Can you work these out from the drawing? Everything is in mm from the part's minimum corner. A direction names the side the tool comes from. Coordinates: 2 decimals unless noted, no trailing zeros. Write each loop counter-clockwise with the first axis right and the second up, starting at its lowest first coordinate (ties: lowest second). Pieces come first, ordered by that corner, then holes. Notation, with made-up numbers: (12, 43.25) -> (64, 43.25) arc R16 ccw to (64, 71.25) -> close; hole circle Ø4 at (4.25, -36). An arc over 180 degrees is marked (long way). Use CSV: the item, a comma, the result in double quotes. Start each with the question number.
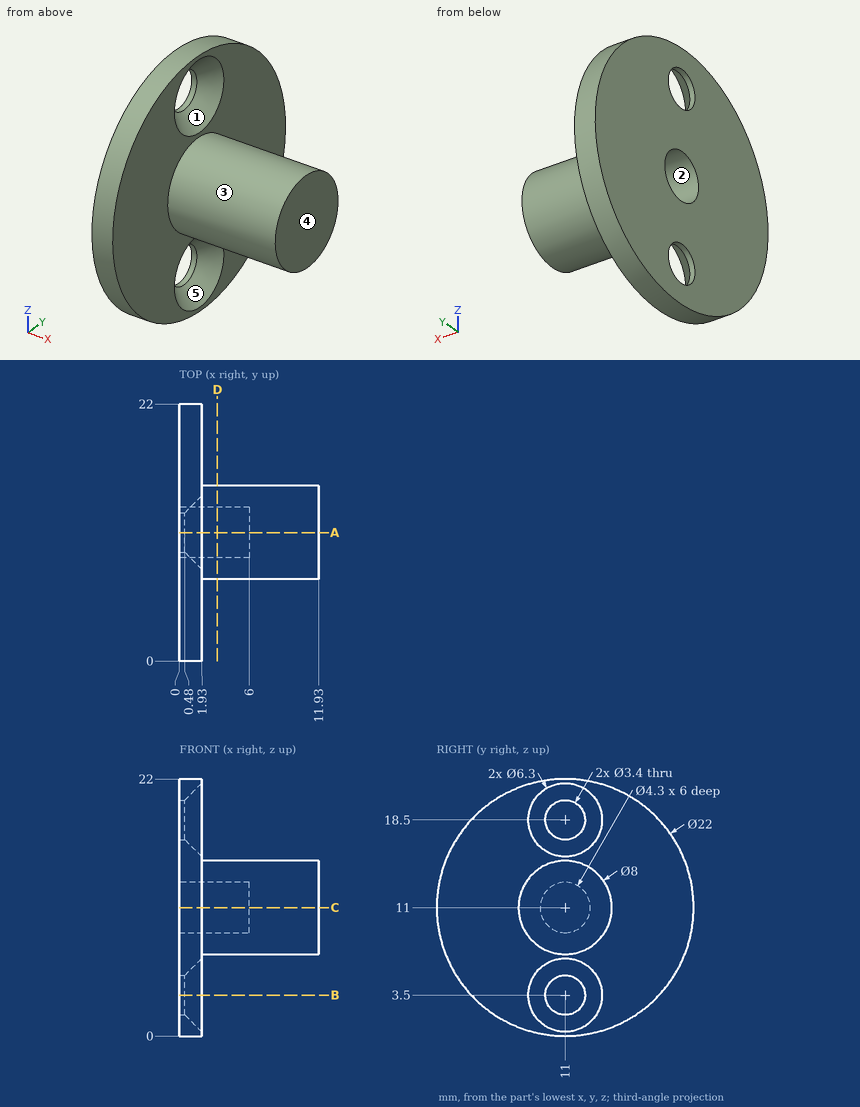
Item 1: Which directions (+Z, -Z, +X, -X, +Y, -Y) give clear straight access to the entire face, cutting with the end or side of a thin tool? Please do the marked faces 1 and 2.
Item 2: I want a section at C-C on z = 11. Please give me the cut outline in (x, y), then the cut area to 3 significant figures.
Item 3: I want a section at B-B on z = 3.5. Please give me the cut outline in (x, y), then the cut area to 3 significant figures.
Item 4: I want a section at D-D on x = 3.25. Please give me the cut outline in (y, z).
Item 5: I want a section at A-A on y = 11. Please give me the cut outline in (x, z), then the cut area to 3 significant figures.
Item 6: I'm going to push flat-ended pins straight in: pin 1 (4 mm diameter, centred on x = 10, z = 17.5, fed in from +Y); pin 2 (6 mm diameter, centred on x = 3, y = 17.5, fed in from -Z); pin 3 (6 mm diameter, centred on x = 5, y = 16.5, fed in from -Z); pin 4 (6 mm diameter, centred on x = 10.5, z = 15, fed in from +Y). Where does each tip first touch, or does it pass through?
Item 7: If I drill on line 1 along Y through (x, z) = (1.8, 11); line 2 along Y through (x, z) = (0.3, 18.5); line 3 along X through (y, z) = (14.5, 18.75), over which ranges is the centre line in solid material (lowest first)?
Item 8: Thinking about a two-plate mould opening in Z: for the marked faces 3, 4 and 5, which applies, +Z half, -Z half, draft (parallel to the pull), parting line (faces both ways), or undercut?
Geometry says:
1,face 1,"+X"
1,face 2,"-X"
2,outline,"(0, 0) -> (1.93, 0) -> (1.93, 7) -> (11.93, 7) -> (11.93, 15) -> (1.93, 15) -> (1.93, 22) -> (0, 22) -> (0, 13.15) -> (6, 13.15) -> (6, 8.85) -> (0, 8.85) -> close"
2,area,"96.7 mm2"
3,outline,"(0, 2.95) -> (1.93, 2.95) -> (1.93, 7.85) -> (0.48, 9.3) -> (0, 9.3) -> close; (0, 12.7) -> (0.48, 12.7) -> (1.93, 14.15) -> (1.93, 19.05) -> (0, 19.05) -> close"
3,area,"22.4 mm2"
4,outline,"circle Ø8 at (11, 11); hole circle Ø4.3 at (11, 11)"
5,outline,"(0, 0) -> (1.93, 0) -> (1.93, 0.35) -> (0.48, 1.8) -> (0, 1.8) -> close; (0, 5.2) -> (0.48, 5.2) -> (1.93, 6.65) -> (1.93, 7) -> (11.93, 7) -> (11.93, 15) -> (1.93, 15) -> (1.93, 15.35) -> (0.48, 16.8) -> (0, 16.8) -> (0, 13.15) -> (6, 13.15) -> (6, 8.85) -> (0, 8.85) -> close; (0, 20.2) -> (0.48, 20.2) -> (1.93, 21.65) -> (1.93, 22) -> (0, 22) -> close"
5,area,"79.3 mm2"
6,pin 1,"through"
6,pin 2,"z = 0.64"
6,pin 3,"z = 7.88"
6,pin 4,"y = 14.87"
7,line 1,"0 to 8.85, 13.15 to 22"
7,line 2,"2.95 to 9.3, 12.7 to 19.05"
7,line 3,"0 to 1.93"
8,face 3,"parting line"
8,face 4,"draft"
8,face 5,"undercut"
